The model under review builds one solid part; all positions refer to its coordinate system, in mm. Give positions to 0.01 mm unless a question says otherwise; leave off trailing zeros. Write each loop counter-clockwise with the first axis right and the second up, starting at its lowest first coordinate (ties: lowest second). Pieces come first, ordered by that corner, then holes. Notation, with made-up numbers: (71, 12.5) - (91, 12.5) arc R16 cw to (91, 41.5) - close; hole circle Ø5 at (23.5, 57.25). An arc over 180 degrees is marked (long way). Write item = value, one per line.
```python
from build123d import *

# Parameters (mm, degrees)
SKETCH1_R           = 10
SKETCH1_R_2         = 7.5
BOSS_EXTRUDE1_DEPTH = 25
THREAD1_PITCH       = 0.3175
SKETCH4_W           = 146
SKETCH4_H           = 146
BOSS_EXTRUDE2_DEPTH = 2
SKETCH5_W           = 148
SKETCH5_H           = 148
BOSS_EXTRUDE3_DEPTH = 1
BOSS_EXTRUDE4_START = 7.5
SKETCH6_W           = 10
SKETCH6_H           = 3
SKETCH6_R           = 1
BOSS_EXTRUDE4_DEPTH = 2.5
BOSS_EXTRUDE5_START = -7.5
SKETCH6_2_W         = 10
SKETCH6_2_H         = 3
SKETCH6_2_R         = 1
BOSS_EXTRUDE5_DEPTH = 2.5
SKETCH9_R           = 18.995637602
CUT_EXTRUDE1_DEPTH  = 111.385687501
CHAMFER1_SIZE       = 3
FILLET1_R           = 1


with BuildPart() as part:
    # Sketch1 → Boss-Extrude1 (new body)
    with BuildSketch(Plane(origin=(0, 0, 0), x_dir=(1, 0, 0), z_dir=(0, 1, 0))):
        with Locations(Location((0, 0, 0), (0, 0, 270))):
            Circle(SKETCH1_R)
        with Locations(Location((0, 0, 0), (0, 0, 270))):
            Circle(SKETCH1_R_2, mode=Mode.SUBTRACT)
    extrude(amount=BOSS_EXTRUDE1_DEPTH)

    # Thread1: the profile of Thread Profile1 profile screwed along a right-hand helix of 18.897638 turns, 6 arcs to a turn; built about Z, then put on its axis
    thread1_z = Axis((0, 0, 0), (0, 0, 1))
    thread1_corners = [(10.0003, 0, -0.000173205), (10.0003, 0, 0.277985704), (9.828148085, 0, 0.17859375), (9.828148085, 0, 0.09921875)]
    with BuildLine(mode=Mode.PRIVATE) as thread1_profile:
        Line(thread1_corners[0], thread1_corners[1])
        Line(thread1_corners[1], thread1_corners[2])
        Line(thread1_corners[2], thread1_corners[3])
        Line(thread1_corners[3], thread1_corners[0])
    thread1_cap = Face(thread1_profile.wire())
    thread1_turn_angles = [0, 30, 60, 90, 120, 150, 180, 210, 240, 270, 300, 330, 360]
    thread1_turn_weights = [1, 0.8660254037844387, 1, 0.8660254037844387, 1, 0.8660254037844387, 1, 0.8660254037844387, 1, 0.8660254037844387, 1, 0.8660254037844387, 1]
    thread1_turn_rails = [Edge.make_bspline([Vector(p[0], p[1], 0).rotate(thread1_z, thread1_turn_angles[k]) / thread1_turn_weights[k] + Vector(0, 0, p[2] + THREAD1_PITCH * thread1_turn_angles[k] / 360) for k in range(13)], [0, 0, 0, 1, 1, 2, 2, 3, 3, 4, 4, 5, 5, 6, 6, 6], 2, thread1_turn_weights) for p in thread1_corners]
    thread1_turn_sides = [Face.make_surface_from_curves(thread1_turn_rails[p[0]], thread1_turn_rails[p[1]]) for p in [(0, 1), (1, 2), (2, 3), (3, 0)]]
    thread1_last_angles = [6480, 6510, 6540, 6570, 6600, 6630, 6660, 6690, 6720, 6750, 6780, 6791.57480315, 6803.149606299]
    thread1_last_weights = [1, 0.8660254037844387, 1, 0.8660254037844387, 1, 0.8660254037844387, 1, 0.8660254037844387, 1, 0.8660254037844387, 1, 0.9796635825089068, 1]
    thread1_last_rails = [Edge.make_bspline([Vector(p[0], p[1], 0).rotate(thread1_z, thread1_last_angles[k]) / thread1_last_weights[k] + Vector(0, 0, p[2] + THREAD1_PITCH * thread1_last_angles[k] / 360) for k in range(13)], [0, 0, 0, 1, 1, 2, 2, 3, 3, 4, 4, 5, 5, 6, 6, 6], 2, thread1_last_weights) for p in thread1_corners]
    thread1_last_sides = [Face.make_surface_from_curves(thread1_last_rails[p[0]], thread1_last_rails[p[1]]) for p in [(0, 1), (1, 2), (2, 3), (3, 0)]]
    thread1 = Plane(origin=(0, -0.5, 0), x_dir=(1, 0, 0), z_dir=(0, 1, 0)) * Solid(Shell([*[p.moved(Location((0, 0, THREAD1_PITCH * i))) for i in range(18) for p in thread1_turn_sides], *thread1_last_sides, thread1_cap, thread1_cap.rotate(thread1_z, 6803.149606299).moved(Location((0, 0, THREAD1_PITCH * 6803.149606299 / 360)))]))
    add(thread1, mode=Mode.SUBTRACT)

    # Sketch4 → Boss-Extrude2 (add)
    with BuildSketch(Plane(origin=(0, 25, 0), x_dir=(1, 0, 0), z_dir=(0, 1, 0))):
        Rectangle(SKETCH4_W, SKETCH4_H)
    extrude(amount=BOSS_EXTRUDE2_DEPTH)

    # Sketch5 → Boss-Extrude3 (add)
    with BuildSketch(Plane.XZ.offset(-25)):
        Rectangle(SKETCH5_W, SKETCH5_H)
    extrude(amount=-BOSS_EXTRUDE3_DEPTH)

    # Sketch6 → Boss-Extrude4 (add, symmetric)
    with BuildSketch(Plane.XY.offset(BOSS_EXTRUDE4_START)):
        with Locations((73, 23.5)):
            Rectangle(SKETCH6_W, SKETCH6_H)
        with Locations((76, 23.5)):
            Circle(SKETCH6_R, mode=Mode.SUBTRACT)
    extrude(amount=BOSS_EXTRUDE4_DEPTH, both=True)

    # Sketch6<2> → Boss-Extrude5 (add, symmetric)
    with BuildSketch(Plane.XY.offset(BOSS_EXTRUDE5_START)):
        with Locations((73, 23.5)):
            Rectangle(SKETCH6_2_W, SKETCH6_2_H)
        with Locations((76, 23.5)):
            Circle(SKETCH6_2_R, mode=Mode.SUBTRACT)
    extrude(amount=BOSS_EXTRUDE5_DEPTH, both=True)

    # Sketch9 → Cut-Extrude1 (cut, through all)
    with BuildSketch(Plane.XZ.offset(-25)):
        Circle(SKETCH9_R)
    extrude(amount=CUT_EXTRUDE1_DEPTH, mode=Mode.SUBTRACT)

    # Chamfer1
    chamfer1_edges = [part.edges().sort_by_distance(p)[0] for p in [
        (68, 25, -7.5),
        (68, 25, 7.5),
    ]]
    chamfer(chamfer1_edges, length=CHAMFER1_SIZE - 0.0001)  # a hair under: the kernel refuses the full size

    # Fillet1
    fillet1_edges = [part.edges().sort_by_distance(p)[0] for p in [
        (78, 22, 7.5),
        (78, 25, 7.5),
        (78, 22, -7.5),
        (78, 25, -7.5),
    ]]
    fillet(fillet1_edges, radius=FILLET1_R)


solid = part.part
```
1. Take a section at A-A on z = -37.5. Give the boundary of the cut face in (x, y), and give its area (3 significant figures).
Findings below:
outline = (-74, 25) - (74, 25) - (74, 26) - (73, 26) - (73, 27) - (-73, 27) - (-73, 26) - (-74, 26) - close
area = 294 mm²
2. For line 1 (Y direction, x = 76, z = 7); line 2 (X direction, y = 25.8, z = -4); line 3 (Z direction, x = -58, y = 26.7), list the stretches that pass through material, from the lowest coordinate up. Write a range as from..to.
Findings below:
line_1 = 22..22.5, 24.5..25
line_2 = -74..74
line_3 = -73..73
3. Take a section at B-B on x = 62. Give the boundary of the cut face in (y, z).
Findings below:
outline = (25, -74) - (26, -74) - (26, -73) - (27, -73) - (27, 73) - (26, 73) - (26, 74) - (25, 74) - close
4. Insertion check: P1, Ø2, axis at y = 26.5, z = 56, coming from the +X side; P2, Ø2.5, axis at x = 71.5, y = 23.5, coming from the +Z side; P3, Ø3.5, axis at x = 75.5, z = -8.5, coming from the +Y side; P4, Ø3, axis at x = 58, y = 23, coming from the -Z side. Each pin has a flat end and moves straight along its axis. Give the tip position at first contact, or say it passes through.
Findings below:
P1 = 74
P2 = 10
P3 = 26
P4 = through
